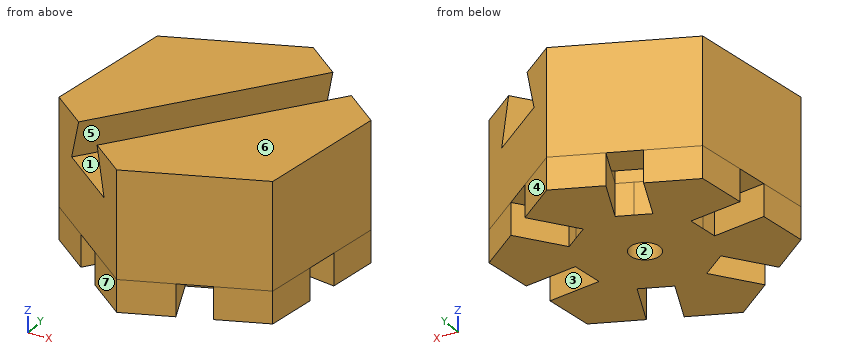
from build123d import *

# Parameters (mm, degrees)
F1_DEPTH = 3
F3_DEPTH = 5
F5_DEPTH = 5
F7_DEPTH = 27.651635
F8_R     = 1.4
F9_DEPTH = 6


with BuildPart() as f1:
    # F0 (on Top) → F1 (new body)
    with BuildSketch(Plane.XY):
        Polygon((5.283907, 9.568716), (1.495191, 12.410254), (-2.859099, 10.550288), (-0.90712, 5.980591), (-2.300426, 5.38543), (-3.689196, 4.782179), (-5.644798, 9.360356), (-10, 7.5), (-10.566367, 2.799092), (-5.632904, 2.204707), (-5.814132, 0.700488), (-5.986087, -0.803848), (-10.928705, -0.20836), (-11.495191, -4.910254), (-7.707268, -7.751196), (-4.725784, -3.775884), (-3.513707, -4.684942), (-2.296891, -5.586028), (-5.283907, -9.568716), (-1.495191, -12.410254), (2.859099, -10.550288), (0.90712, -5.980591), (2.300426, -5.38543), (3.689196, -4.782179), (5.644798, -9.360356), (10, -7.5), (10.566367, -2.799092), (5.632904, -2.204707), (5.814132, -0.700488), (5.986087, 0.803848), (10.928705, 0.20836), (11.495191, 4.910254), (7.707268, 7.751196), (4.725784, 3.775884), (3.513707, 4.684942), (2.296891, 5.586028), align=None)
    extrude(amount=F1_DEPTH)

    # F2 (on face) → F3 (join)
    with BuildSketch(Plane.XY.offset(3)):
        Polygon((-10, 7.5), (-11.495191, -4.910254), (-1.495191, -12.410254), (10, -7.5), (11.495191, 4.910254), (1.495191, 12.410254), align=None)
        Polygon((-2.296891, -5.586028), (-3.496891, -7.186028), (-5.920251, -5.368507), (-4.725784, -3.775884), align=None, mode=Mode.SUBTRACT)
        Polygon((3.689196, -4.782179), (4.474837, -6.62141), (1.689138, -7.811341), (0.90712, -5.980591), align=None, mode=Mode.SUBTRACT)
        Polygon((5.986087, 0.803848), (7.971728, 0.564618), (7.609389, -2.442834), (5.632904, -2.204707), align=None, mode=Mode.SUBTRACT)
        Polygon((-5.986087, -0.803848), (-7.971728, -0.564618), (-7.609389, 2.442834), (-5.632904, 2.204707), align=None, mode=Mode.SUBTRACT)
        Polygon((-3.689196, 4.782179), (-4.474837, 6.62141), (-1.689138, 7.811341), (-0.90712, 5.980591), align=None, mode=Mode.SUBTRACT)
        Polygon((2.296891, 5.586028), (3.496891, 7.186028), (5.920251, 5.368507), (4.725784, 3.775884), align=None, mode=Mode.SUBTRACT)
    extrude(amount=F3_DEPTH)

    # F4 (on face) → F5 (join)
    with BuildSketch(Plane.XY.offset(8)):
        Polygon((-11.495191, -4.910254), (-1.495191, -12.410254), (10, -7.5), (11.495191, 4.910254), (1.495191, 12.410254), (-10, 7.5), align=None)
    extrude(amount=F5_DEPTH)

    # F6 (on face) → F7 (cut, through all)
    with BuildSketch(Plane(origin=(-6.495191, -8.660254, 0), x_dir=(0.8, -0.6, 0), z_dir=(-0.6, -0.8, 0))):
        Polygon((-3.5, 9), (3.5, 9), (2, 13), (-2, 13), align=None)
    extrude(amount=-F7_DEPTH, mode=Mode.SUBTRACT)

    # F8 (on face) → F9 (cut)
    with BuildSketch(Plane(origin=(0, 0, 0), x_dir=(1, 0, 0), z_dir=(0, 0, -1))):
        Circle(F8_R)
    extrude(amount=-F9_DEPTH, mode=Mode.SUBTRACT)


solid = f1.part
Source: CAD feature listing. Evaluate the final solid. Frame: model axes, mm. Face numbers are marked on the shaded views. A direction names the side the tool comes from. Coordinates: 2 decimals unless noted, no trailing zeros. Order: outer loops, then holes, each group sorted by start corner. A loop starts at its lowest first (then second) coordinate and runs counter-clockwise, first axis right, second up.
Item 1: First-contact query: P1, Ø4, axis at x = 7, z = 9.5, coming from the +Y side; P2, Ø1.4, axis at x = 3, y = 5, coming from the +Z side; P3, Ø2.5, axis at x = -3, y = 7, coming from the -Z side. Flat tips, straight axial feed; report the tip coordinate or a pass-through.
Output values:
P1: stops at y = 9.73
P2: stops at z = 9
P3: stops at z = 3
Item 2: Set-up query: the marked faces 1, 2 and 3. Return all of +Z, -Z, +X, -X, +Y, -Y with unobstructed straight access to the full face (end or side cutting, diameter ignored); none if empty.
Output values:
face 1: none
face 2: -Z
face 3: -Z, +X
Item 3: Material intervals for line 1 (Y direction, x = 2.75, z = 3.5); line 2 (X direction, y = 0, z = 4.05); line 3 (Z direction, x = -1, y = -2.5), sorted ascending.
Output values:
line 1: y = -10.6 to -7.36, -5.19 to 5.25, 6.19 to 11.47
line 2: x = -10.9 to -7.9, -5.89 to -1.4, 1.4 to 5.89, 7.9 to 10.9
line 3: z = 0 to 9
Item 4: Cut plane A-A (z = 5). Count the separate pieces of the cut face and the enclosed holes in it, plus the area to 3 significant figures.
Output values:
separate pieces: 1
enclosed holes: 7
area: 364 mm2
Item 5: Pull-direction query (X, two-part tool) for the marked faces 4, 5, 6 and 7; classes: pulls with the +X half, pulls with the -X half, needs draft (parallel to the pull), parting line crosses it, or undercut.
Output values:
face 4: pulls with the +X half
face 5: undercut
face 6: needs draft
face 7: pulls with the -X half
Item 6: Cut plane D-D (y = -3.25). Return loops of the section in (x, z).
Output values:
outline: (-11.3, 0) - (10.51, 0) - (10.51, 13) - (0.06, 13) - (1.94, 9) - (-6.81, 9) - (-4.94, 13) - (-11.3, 13) - close
Item 7: Cut plane C-C (x = 0). Return loops of the section in (y, z).
Output values:
outline: (-11.77, 0) - (-1.4, 0) - (-1.4, 6) - (1.4, 6) - (1.4, 0) - (11.77, 0) - (11.77, 13) - (3.33, 13) - (5.83, 9) - (-5.83, 9) - (-3.33, 13) - (-11.77, 13) - close
Item 8: Cut plane B-B (z = 9.5). Return loops of the section in (x, y), plus the area to 3 significant figures.
Output values:
outline: (-11.5, -4.91) - (-9.15, -6.67) - (3.85, 10.65) - (1.5, 12.41) - (-10, 7.5) - close; (-3.85, -10.65) - (-1.5, -12.41) - (10, -7.5) - (11.5, 4.91) - (9.15, 6.67) - close
area: 263 mm2
